from build123d import *

# Parameters (mm, degrees)
SKETCH1_W           = 101.6
SKETCH1_H           = 50.8
BOSS_EXTRUDE1_DEPTH = 1219.2
SKETCH2_W           = 101.6
SKETCH2_H           = 50.8
CUT_EXTRUDE1_DEPTH  = 101.6
SKETCH3_W           = 50.8
SKETCH3_H           = 50.8
CUT_EXTRUDE2_DEPTH  = 50.8


with BuildPart() as part:
    # Sketch1 → Boss-Extrude1 (new body)
    with BuildSketch(Plane.XY):
        Rectangle(SKETCH1_W, SKETCH1_H)
    extrude(amount=BOSS_EXTRUDE1_DEPTH)

    # Sketch2 → Cut-Extrude1 (cut)
    with BuildSketch(Plane.XY.offset(1219.2)):
        Rectangle(SKETCH2_W, SKETCH2_H)
    extrude(amount=-CUT_EXTRUDE1_DEPTH, mode=Mode.SUBTRACT)

    # Sketch3 → Cut-Extrude2 (cut)
    with BuildSketch(Plane.ZY.offset(50.8)):
        with Locations((1066.8, 0)):
            Rectangle(SKETCH3_W, SKETCH3_H)
    extrude(amount=-CUT_EXTRUDE2_DEPTH, mode=Mode.SUBTRACT)


solid = part.part
Read the model definition and answer for the solid it produces. Units are mm, in the model's axes. A direction names the side the tool comes from. Give positions to 0.01 mm unless a question says otherwise; leave off trailing zeros. Write each loop counter-clockwise with the first axis right and the second up, starting at its lowest first coordinate (ties: lowest second). Pieces come first, ordered by that corner, then holes. Notation, with made-up numbers: M 24,57.5 L 42,57.5 A20 ccw 42,84.5 Z; hole C -37.5,59.25 d9. An arc over 180 degrees is marked long. One line per item, written item: value. Start each with the question number.
(1) Determine the mould class of faces 3 (the flat face through (0, 0, 1066)), 4 (the flat face through (-1, 0, 0)), 5 (the flat face through (-1, 0, 1117.6)), 6 (the flat face through (-1, 25.4, 551)) for opening direction Z: pulls with the +Z half, pulls with the -Z half, needs draft (parallel to the pull), parting line crosses it, or undercut.
(2) Find section B-B (y = -12). Determine the outline of the cut face in (x, z).
(3) Find section A-A (x = -21). Determine the outline of the cut face in (y, z), plus the area to 3 significant figures.
(4) Find the intervals of material crossed by line 1 (Z direction, x = -24, y = 2), in increasing order.
(5) A tool of negligible diameter and unlimited length cuts with its end or side. For faces 1 (the flat face through (-50.8, 0, 513)), 2 (the flat face through (-26, 0, 1092.2)), from which of +Z, -Z, +X, -X, +Y, -Y can it reach the whole face along a straight path? Write none if from no direction.
Results below:
1. face 3: undercut
1. face 4: pulls with the -Z half
1. face 5: pulls with the +Z half
1. face 6: needs draft
2. outline: M -50.8,0 L 50.8,0 L 50.8,1117.6 L -50.8,1117.6 L -50.8,1092.2 L 0,1092.2 L 0,1041.4 L -50.8,1041.4 Z
3. outline: M -25.4,0 L 25.4,0 L 25.4,1041.4 L -25.4,1041.4 Z; M -25.4,1092.2 L 25.4,1092.2 L 25.4,1117.6 L -25.4,1117.6 Z
3. area: 54,200 mm^2
4. line 1: z = 0 to 1041.4, 1092.2 to 1117.6
5. face 1: +Z, -Z, -X, +Y, -Y
5. face 2: -X, +Y, -Y
